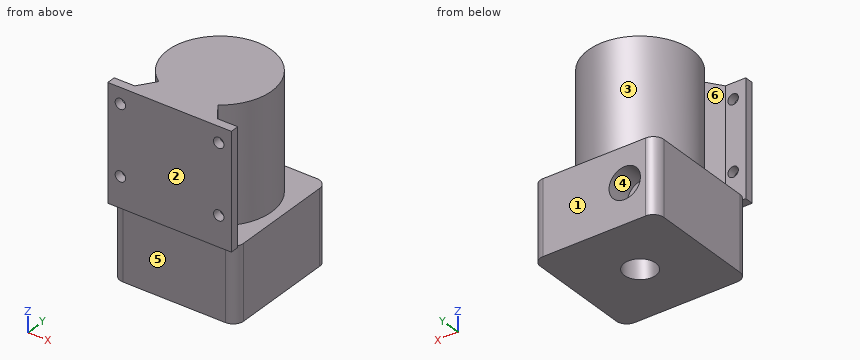
Autodesk Inventor part; units mm, degrees
ref_plane "YZ Plane" through (0, 0, 0) normal (1, 0, 0) x (0, 1, 0)
ref_plane "XZ Plane" through (0, 0, 0) normal (0, 1, 0) x (-1, 0, 0)
ref_plane "XY Plane" through (0, 0, 0) normal (0, 0, 1) x (1, 0, 0)
sketch "Sketch1" plane through (0, 0, 0) normal (0, 0, 1) x (1, 0, 0)
  line L0 (0, 0) -> (50, 0)
  line L1 (50, 0) -> (50, 50)
  line L2 (50, 50) -> (0, 50)
  line L3 (0, 50) -> (0, 0)
  line L4 (5.3353, 5.3353) -> (44.6647, 5.3353) construction
  line L5 (44.6647, 5.3353) -> (44.6647, 44.6647) construction
  line L6 (44.6647, 44.6647) -> (5.3353, 44.6647) construction
  line L7 (5.3353, 44.6647) -> (5.3353, 5.3353) construction
  line L8 (25, 44.6647) -> (25, 50) construction
  line L9 (44.6647, 25) -> (50, 25) construction
  dimension "d0" = 50
extrude "Extrusion1" add sketch "Sketch1" along normal blind 30
sketch "Sketch2" plane through (0, 0, 30) normal (0, 0, 1) x (1, 0, 0)
  line L0 (0, -2.5) -> (50, -2.5)
  line L1 (50, -2.5) -> (50, 1)
  line L2 (50, 1) -> (0, 1)
  line L3 (0, 1) -> (0, -2.5)
  circle A0 centre (25, 25) radius 21
  line L4 (50, 50) -> (0, 50) construction
  line L5 (50, 0) -> (50, 50) construction
  line L6 (25, 25) -> (25, 50) construction
  line L7 (25, 25) -> (50, 25) construction
  line L8 (13, 7.7663) -> (37, 7.7663)
  line L9 (8.2885, 1) -> (25, 25)
  line L10 (25, 25) -> (41.7115, 1)
  point P0 (0, 0)
  point P1 (0, -0.75)
  point P2 (50, -0.75)
  dimension "d3" = 2.5
  dimension "d4" = 3.5
  dimension "d5" = 42
  dimension "d6" = 24
extrude "Extrusion2" add sketch "Sketch2" along normal blind 46.5
sketch "Sketch3" plane through (0, -2.5, 30) normal (0, -1, 0) x (1, 0, 0)
  line L0 (44.8967, 40.15) -> (5.1033, 40.15) construction
  line L1 (5.1033, 40.15) -> (5.1033, 12.21) construction
  line L2 (5.1033, 12.21) -> (44.8967, 12.21) construction
  line L3 (44.8967, 12.21) -> (44.8967, 40.15) construction
  line L4 (0, 46.5) -> (50, 46.5) construction
  line L5 (25, 40.15) -> (25, 46.5) construction
  circle A0 centre (44.8967, 40.15) radius 2.1167
  circle A1 centre (44.8967, 12.21) radius 2.1167
  circle A2 centre (5.1033, 40.15) radius 2.1167
  circle A3 centre (5.1033, 12.21) radius 2.1167
  point P0 (0, -30)
  dimension "d9" = 27.94
  dimension "d10" = 6.35
  dimension "d11" = 39.7933
  dimension "d12" = 4.2333
extrude "Extrusion3" cut sketch "Sketch3" against normal up to surface (3.5 mm away)
sketch "Sketch4" plane through (0, 0, 0) normal (0, 0, -1) x (-1, 0, 0)
  circle A0 centre (-25, 25) radius 6.35
  line L0 (-50, 50) -> (0, 50) construction
  line L1 (0, 50) -> (0, 0) construction
  point P0 (-25, 50)
  point P1 (0, 25)
  dimension "d15" = 12.7
extrude "Extrusion4" cut sketch "Sketch4" against normal blind 10
sketch "Sketch5" plane through (0, 50, 0) normal (0, 1, 0) x (1, 0, 0)
  circle A0 centre (12.7, -15.875) radius 6.35
  point P0 (0, 0)
  dimension "d18" = 12.7
  dimension "d19" = 12.7
  dimension "d20" = 15.875
extrude "Extrusion5" cut sketch "Sketch5" against normal blind 10
fillet "Fillet1" radius 4.2333 4 edges at (50, 50, 15) (0, 50, 15) (0, 0, 15) (50, 0, 15)
properties part number "Water_pump"
Geometry: final body of the model. Coordinates: model frame, mm. Face numbers are marked on the shaded views. A direction names the side the tool comes from. Give positions to 0.01 mm unless a question says otherwise; leave off trailing zeros. Loops run counter-clockwise (first coordinate to the right, second up) from the corner with the lowest first, then second, coordinate; pieces in that order, holes last. Notation, with made-up numbers: (-29.5, -30) -> (18.5, -30) arc R25 ccw to (18.5, -2) -> close; hole circle Ø6 at (42.25, 75.25). An arc over 180 degrees is marked (long way). Put each result on its own line as item: value.
1. Ray query, line 1 along X through (y, z) = (-1, 42); line 2 along Y through (x, z) = (22, 26); line 3 along Y through (x, z) = (22, 66.5). Return the intervals inside material, ascending. Write a range as [from, to].
Taken from the geometry:
line 1: x = [0, 3], [7.21, 42.79], [47, 50]
line 2: y = [0, 50]
line 3: y = [-2.5, 45.78]
2. Cut plane A-A (z = 70.15). Return the cut outline in (x, y), plus the area to 3 significant figures.
Taken from the geometry:
outline: (0, -2.5) -> (2.99, -2.5) -> (2.99, 1) -> (0, 1) -> close; (7.22, -2.5) -> (42.78, -2.5) -> (42.78, 1) -> (41.71, 1) -> (37, 7.77) arc R21 ccw (long way) to (13, 7.77) -> (8.29, 1) -> (7.22, 1) -> close; (47.01, -2.5) -> (50, -2.5) -> (50, 1) -> (47.01, 1) -> close
area: 1,660 mm2
3. Pull-direction query (Y, two-part tool) for the marked faces 1, 2 and 3; classes: released by +Y, released by -Y, zero draft, split by the parting line, or undercut.
Taken from the geometry:
face 1: released by +Y
face 2: released by -Y
face 3: undercut
4. Set-up query: the marked faces 4, 5 and 6. Return all of +Z, -Z, +X, -X, +Y, -Y with unobstructed straight access to the full face (end or side cutting, diameter ignored); none if empty.
Taken from the geometry:
face 4: +Y
face 5: -Z, +X, -X, -Y
face 6: +Z, -X
5. Cut plane C-C (x = 25). Return the cut outline in (y, z).
Taken from the geometry:
outline: (-2.5, 30) -> (0, 30) -> (0, 0) -> (18.65, 0) -> (18.65, 10) -> (31.35, 10) -> (31.35, 0) -> (50, 0) -> (50, 30) -> (46, 30) -> (46, 76.5) -> (-2.5, 76.5) -> close
6. Pin query (flat end, axial travel): P1, Ø6, axis at y = 10.5, z = 35.5, coming from the +X side; P2, Ø5.5, axis at x = 5.1, z = 70.15, coming from the +Y side; P3, Ø5, axis at x = 36.5, z = 50, coming from the +Y side; P4, Ø3, axis at y = 34.5, z = 28, coming from the -X side. Return the tip coordinate at first contact, or that it passes through.
Taken from the geometry:
P1: stops at x = 42.57
P2: stops at y = 37.12
P3: stops at y = 43.97
P4: stops at x = 0
7. Cut plane B-B (z = 26). Return the cut outline in (x, y), plus the area to 3 significant figures.
Taken from the geometry:
outline: (0, 4.23) arc R4.23 ccw to (4.23, 0) -> (45.77, 0) arc R4.23 ccw to (50, 4.23) -> (50, 45.77) arc R4.23 ccw to (45.77, 50) -> (4.23, 50) arc R4.23 ccw to (0, 45.77) -> close
area: 2,480 mm2
8. Cut plane D-D (y = 38). Return the cut outline in (x, z).
Taken from the geometry:
outline: (0, 0) -> (50, 0) -> (50, 30) -> (41.49, 30) -> (41.49, 76.5) -> (8.51, 76.5) -> (8.51, 30) -> (0, 30) -> close
